Check sheet for the drawn part. Datum: minimum x, y, z corner. Units: mm. Round coordinates to 2 decimals unless told otherwise and drop trailing zeros. Loops run counter-clockwise (first coordinate to the right, second up) from the corner with the lowest first, then second, coordinate; pieces in that order, holes last.
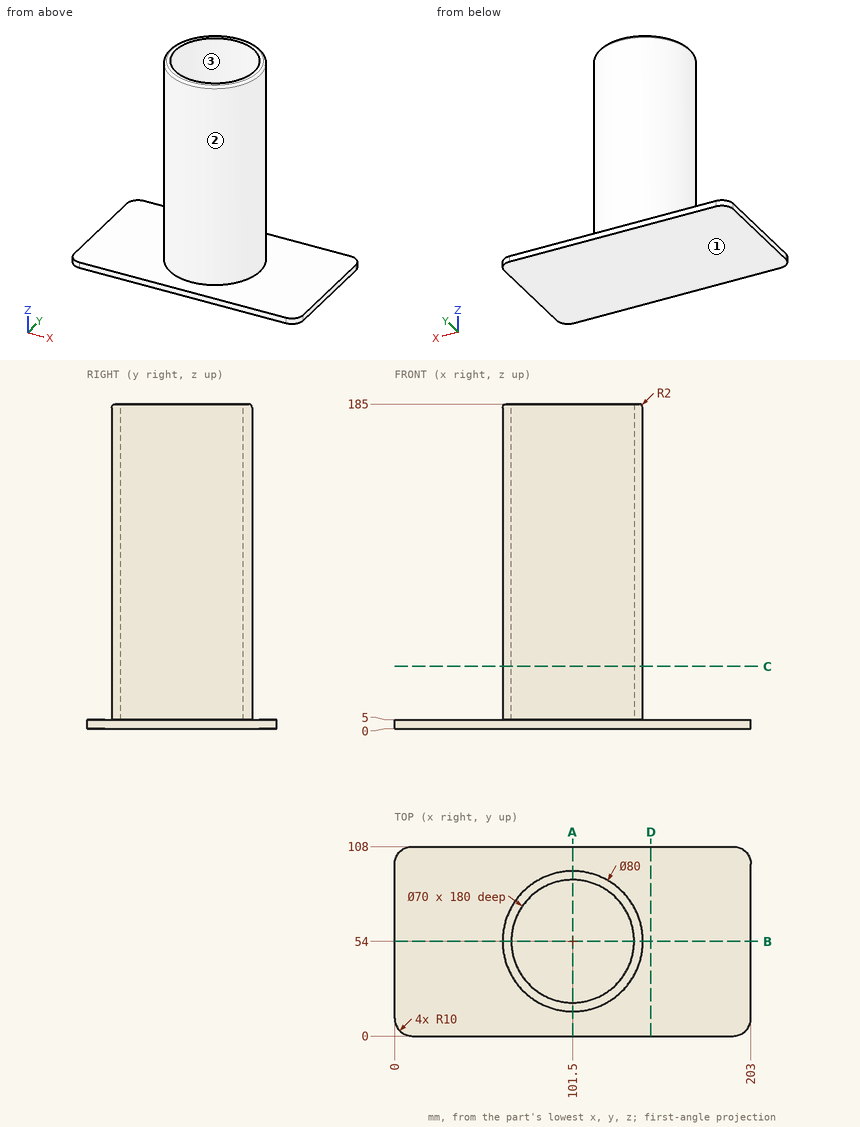
1) Sectioned sample at A-A, the plane x = 101.5. Record the cut outline in (y, z).
Report:
outline: (0, 0) - (108, 0) - (108, 5) - (94, 5) - (94, 183) arc R2 ccw to (92, 185) - (89, 185) - (89, 5) - (19, 5) - (19, 185) - (16, 185) arc R2 ccw to (14, 183) - (14, 5) - (0, 5) - close
2) Scan lines: line 1 along Y through (x, z) = (101, 94); line 2 along Z through (x, y) = (83.5, 65); line 3 along X through (y, z) = (67, 64). Record each from-to range of solid material in increasing order.
Report:
line 1: y = 14 to 19, 89 to 94
line 2: z = 0 to 5
line 3: x = 63.67 to 69, 134 to 139.33
3) Mould release check, pull along X, two halves, no side actions. Record for the marked faces 1, 2 and 3: +X half, -X half, draft (parallel to the pull), parting line (faces both ways), or undercut.
Report:
face 1: draft
face 2: parting line
face 3: undercut
4) Sectioned sample at B-B, the plane y = 54. Record the cut outline in (x, z), then the cut area to 3 significant figures.
Report:
outline: (0, 0) - (203, 0) - (203, 5) - (141.5, 5) - (141.5, 183) arc R2 ccw to (139.5, 185) - (136.5, 185) - (136.5, 5) - (66.5, 5) - (66.5, 185) - (63.5, 185) arc R2 ccw to (61.5, 183) - (61.5, 5) - (0, 5) - close
area: 2,810 mm2
5) Sectioned sample at C-C, the plane z = 35.5. Record the cut outline in (x, y), then the cut area to 3 significant figures.
Report:
outline: circle Ø80 at (101.5, 54); hole circle Ø70 at (101.5, 54)
area: 1,180 mm2
6) Sectioned sample at D-D, the plane x = 146. Record the cut outline in (y, z), then the cut area to 3 significant figures.
Report:
outline: (0, 0) - (108, 0) - (108, 5) - (0, 5) - close
area: 540 mm2
7) Gauge pin test, flat ends, axial feed: pin 1 (21 mm diameter, centred on x = 103, y = 52.5, fed in from +Z); pin 2 (1 mm diameter, centred on y = 61.5, z = 95.5, fed in from -X); pin 3 (2 mm diameter, centred on x = 69.5, z = 160, fed in from +Y). Record the tip position at first contact, or that the pin passes through.
Report:
pin 1: stops at z = 5
pin 2: stops at x = 62.12
pin 3: stops at y = 79.28
